Can you work these out from the model? Positions are in its coordinate system, mm. Coordinates: 2 decimals unless noted, no trailing zeros. Write each loop counter-clockwise with the first axis right and the second up, starting at its lowest first coordinate (ties: lowest second). Pieces come first, ordered by that corner, then holes. Notation, with made-up numbers: M 6,23.25 L 15,23.25 A33 cw 15,60.25 Z; hole C -11,39 d8. An arc over 180 degrees is marked long. Use one line per item in the form item = value. Start each with the question number.
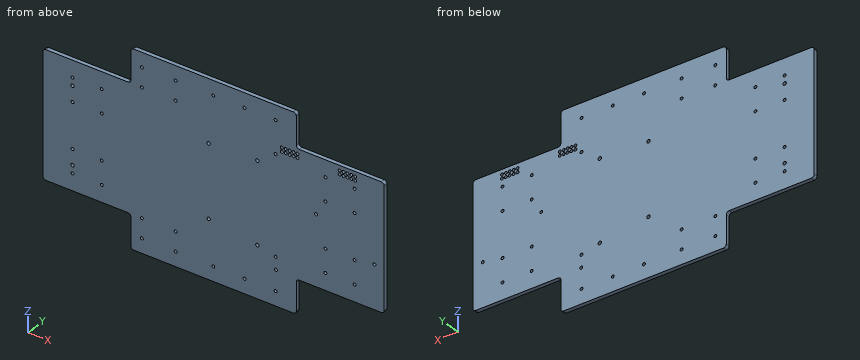
```python
from build123d import *

# Parameters (mm, degrees)
SKETCH_1_R          = 1.75
SKETCH_1_R_2        = 1.5
EXTRUDE_1_DEPTH     = 4
SKETCH_2_R          = 1.5
CUT_EXTRUDE_1_DEPTH = 5
FILLET_1_R          = 3
FILLET_2_R          = 3
FILLET_3_R          = 3
FILLET_4_R          = 3
FILLET_5_R          = 3
FILLET_6_R          = 3
FILLET_7_R          = 3
FILLET_8_R          = 3
FILLET_9_R          = 3
FILLET_10_R         = 3
FILLET_11_R         = 3
FILLET_12_R         = 3
SKETCH_3_R          = 1.75
CUT_EXTRUDE_2_DEPTH = 5
SKETCH_5_R          = 1.5
CUT_EXTRUDE_3_DEPTH = 5
SKETCH_6_R          = 1.5
CUT_EXTRUDE_4_DEPTH = 10


with BuildPart() as part:
    # 草图1 → 凸台-拉伸1 (new body)
    with BuildSketch(Plane(origin=(0, 0, 0), x_dir=(1, 0, 0), z_dir=(0, 1, 0))):
        Polygon((-165.354330709, -0.523412356), (-165.354330709, 129.476587644), (-75.154330709, 129.476587644), (-75.154330709, 164.476587644), (94.445669291, 164.476587644), (94.445669291, 129.476587644), (184.645669291, 129.476587644), (184.645669291, -0.523412356), (94.445669291, -0.523412356), (94.445669291, -35.523412356), (-75.154330709, -35.523412356), (-75.154330709, -0.523412356), align=None)
        with Locations((-135.060351007, 24.855830169)):
            Circle(SKETCH_1_R, mode=Mode.SUBTRACT)
        with Locations((-135.060351007, 104.097345119)):
            Circle(SKETCH_1_R, mode=Mode.SUBTRACT)
        with Locations((-105.060351007, 87.897345119)):
            Circle(SKETCH_1_R_2, mode=Mode.SUBTRACT)
        with Locations((-105.060351007, 112.097345119)):
            Circle(SKETCH_1_R_2, mode=Mode.SUBTRACT)
        with Locations((-135.060351007, 87.897345119)):
            Circle(SKETCH_1_R_2, mode=Mode.SUBTRACT)
        with Locations((-135.060351007, 112.097345119)):
            Circle(SKETCH_1_R_2, mode=Mode.SUBTRACT)
        with Locations((-105.060351007, 41.055830169)):
            Circle(SKETCH_1_R_2, mode=Mode.SUBTRACT)
        with Locations((-135.060351007, 41.055830169)):
            Circle(SKETCH_1_R_2, mode=Mode.SUBTRACT)
        with Locations((-105.060351007, 16.855830169)):
            Circle(SKETCH_1_R_2, mode=Mode.SUBTRACT)
        with Locations((-135.060351007, 16.855830169)):
            Circle(SKETCH_1_R_2, mode=Mode.SUBTRACT)
        with Locations((124.351689589, 16.855830169)):
            Circle(SKETCH_1_R_2, mode=Mode.SUBTRACT)
        with Locations((154.351689589, 16.855830169)):
            Circle(SKETCH_1_R_2, mode=Mode.SUBTRACT)
        with Locations((124.351689589, 41.055830169)):
            Circle(SKETCH_1_R_2, mode=Mode.SUBTRACT)
        with Locations((154.351689589, 41.055830169)):
            Circle(SKETCH_1_R_2, mode=Mode.SUBTRACT)
        with Locations((124.351689589, 87.897345119)):
            Circle(SKETCH_1_R_2, mode=Mode.SUBTRACT)
        with Locations((154.351689589, 87.897345119)):
            Circle(SKETCH_1_R_2, mode=Mode.SUBTRACT)
        with Locations((124.351689589, 112.097345119)):
            Circle(SKETCH_1_R_2, mode=Mode.SUBTRACT)
        with Locations((154.351689589, 112.097345119)):
            Circle(SKETCH_1_R_2, mode=Mode.SUBTRACT)
    extrude(amount=EXTRUDE_1_DEPTH)

    # 草图2 → 切除-拉伸1 (cut, through all)
    with BuildSketch(Plane(origin=(0, 4, 0), x_dir=(1, 0, 0), z_dir=(0, 1, 0))):
        with Locations((-29.350172185, 149.476587644)):
            Circle(SKETCH_2_R)
        with Locations((-29.350172185, 129.476587644)):
            Circle(SKETCH_2_R)
        with Locations((-63.922255051, 149.476587644)):
            Circle(SKETCH_2_R)
        with Locations((-63.922255051, 129.476587644)):
            Circle(SKETCH_2_R)
        with Locations((-29.350172185, -0.523412356)):
            Circle(SKETCH_2_R)
        with Locations((-29.350172185, -20.523412356)):
            Circle(SKETCH_2_R)
        with Locations((-63.922255051, -20.523412356)):
            Circle(SKETCH_2_R)
        with Locations((-63.922255051, -0.523412356)):
            Circle(SKETCH_2_R)
        with Locations((9.288549374, 149.476587644)):
            Circle(SKETCH_2_R)
        with Locations((41.288549374, 149.476587644)):
            Circle(SKETCH_2_R)
        with Locations((73.288549374, 149.476587644)):
            Circle(SKETCH_2_R)
        with Locations((73.288549374, 115.508346765)):
            Circle(SKETCH_2_R)
        with Locations((41.288549374, -20.523412356)):
            Circle(SKETCH_2_R)
        with Locations((73.288549374, -20.523412356)):
            Circle(SKETCH_2_R)
        with Locations((73.288549374, 13.444828523)):
            Circle(SKETCH_2_R)
        with Locations((9.288549374, -20.523412356)):
            Circle(SKETCH_2_R)
    extrude(amount=-CUT_EXTRUDE_1_DEPTH, mode=Mode.SUBTRACT)

    # 圆角1
    fillet_1_edges = [part.edges().sort_by_distance(p)[0] for p in [
        (-75.154330709, 2, -164.476587644),
    ]]
    fillet(fillet_1_edges, radius=FILLET_1_R)

    # 圆角2
    fillet_2_edges = [part.edges().sort_by_distance(p)[0] for p in [
        (-165.354330709, 2, -129.476587644),
    ]]
    fillet(fillet_2_edges, radius=FILLET_2_R)

    # 圆角3
    fillet_3_edges = [part.edges().sort_by_distance(p)[0] for p in [
        (-75.154330709, 2, -129.476587644),
    ]]
    fillet(fillet_3_edges, radius=FILLET_3_R)

    # 圆角4
    fillet_4_edges = [part.edges().sort_by_distance(p)[0] for p in [
        (-165.354330709, 2, 0.523412356),
    ]]
    fillet(fillet_4_edges, radius=FILLET_4_R)

    # 圆角5
    fillet_5_edges = [part.edges().sort_by_distance(p)[0] for p in [
        (-75.154330709, 2, 0.523412356),
    ]]
    fillet(fillet_5_edges, radius=FILLET_5_R)

    # 圆角6
    fillet_6_edges = [part.edges().sort_by_distance(p)[0] for p in [
        (-75.154330709, 2, 35.523412356),
    ]]
    fillet(fillet_6_edges, radius=FILLET_6_R)

    # 圆角7
    fillet_7_edges = [part.edges().sort_by_distance(p)[0] for p in [
        (94.445669291, 2, 35.523412356),
    ]]
    fillet(fillet_7_edges, radius=FILLET_7_R)

    # 圆角8
    fillet_8_edges = [part.edges().sort_by_distance(p)[0] for p in [
        (94.445669291, 2, 0.523412356),
    ]]
    fillet(fillet_8_edges, radius=FILLET_8_R)

    # 圆角9
    fillet_9_edges = [part.edges().sort_by_distance(p)[0] for p in [
        (184.645669291, 2, 0.523412356),
    ]]
    fillet(fillet_9_edges, radius=FILLET_9_R)

    # 圆角10
    fillet_10_edges = [part.edges().sort_by_distance(p)[0] for p in [
        (184.645669291, 2, -129.476587644),
    ]]
    fillet(fillet_10_edges, radius=FILLET_10_R)

    # 圆角11
    fillet_11_edges = [part.edges().sort_by_distance(p)[0] for p in [
        (94.445669291, 2, -129.476587644),
    ]]
    fillet(fillet_11_edges, radius=FILLET_11_R)

    # 圆角12
    fillet_12_edges = [part.edges().sort_by_distance(p)[0] for p in [
        (94.445669291, 2, -164.476587644),
    ]]
    fillet(fillet_12_edges, radius=FILLET_12_R)

    # 草图3 → 切除-拉伸2 (cut, through all)
    with BuildSketch(Plane(origin=(0, 4, 0), x_dir=(1, 0, 0), z_dir=(0, 1, 0))):
        with Locations((54.598317565, 26.976587644)):
            Circle(SKETCH_3_R)
        with Locations((54.598317565, 110.976587644)):
            Circle(SKETCH_3_R)
        with Locations((4.598317565, 28.976587644)):
            Circle(SKETCH_3_R)
        with Locations((4.598317565, 103.976587644)):
            Circle(SKETCH_3_R)
    extrude(amount=-CUT_EXTRUDE_2_DEPTH, mode=Mode.SUBTRACT)

    # 草图5 → 切除-拉伸3 (cut, through all)
    with BuildSketch(Plane(origin=(0, 4, 0), x_dir=(1, 0, 0), z_dir=(0, 1, 0))):
        with Locations((73.645669291, 128.296587644)):
            Circle(SKETCH_5_R)
        with Locations((174.645669291, 84.296587644)):
            Circle(SKETCH_5_R)
        with Locations((114.645669291, 57.296587644)):
            Circle(SKETCH_5_R)
    extrude(amount=-CUT_EXTRUDE_3_DEPTH, mode=Mode.SUBTRACT)

    # 草图6 → 切除-拉伸4 (cut)
    with BuildSketch(Plane(origin=(0, 4, 0), x_dir=(1, 0, 0), z_dir=(0, 1, 0))):
        with Locations((146.895669291, 8.486587644)):
            Circle(SKETCH_6_R)
        with Locations((83.635669291, 8.486587644)):
            Circle(SKETCH_6_R)
        with Locations((142.895669291, 8.486587644)):
            Circle(SKETCH_6_R)
        with Locations((79.635669291, 8.486587644)):
            Circle(SKETCH_6_R)
        with Locations((138.895669291, 8.486587644)):
            Circle(SKETCH_6_R)
        with Locations((87.635669291, 8.486587644)):
            Circle(SKETCH_6_R)
        with Locations((91.635669291, 8.486587644)):
            Circle(SKETCH_6_R)
        with Locations((150.895669291, 8.486587644)):
            Circle(SKETCH_6_R)
        with Locations((95.635669291, 8.486587644)):
            Circle(SKETCH_6_R)
        with Locations((154.895669291, 8.486587644)):
            Circle(SKETCH_6_R)
        with Locations((87.635669291, 4.486587644)):
            Circle(SKETCH_6_R)
        with Locations((146.895669291, 4.486587644)):
            Circle(SKETCH_6_R)
        with Locations((79.635669291, 4.486587644)):
            Circle(SKETCH_6_R)
        with Locations((83.635669291, 4.486587644)):
            Circle(SKETCH_6_R)
        with Locations((91.635669291, 4.486587644)):
            Circle(SKETCH_6_R)
        with Locations((95.635669291, 4.486587644)):
            Circle(SKETCH_6_R)
        with Locations((138.895669291, 4.486587644)):
            Circle(SKETCH_6_R)
        with Locations((142.895669291, 4.486587644)):
            Circle(SKETCH_6_R)
        with Locations((150.895669291, 4.486587644)):
            Circle(SKETCH_6_R)
        with Locations((154.895669291, 4.486587644)):
            Circle(SKETCH_6_R)
    extrude(amount=-CUT_EXTRUDE_4_DEPTH, mode=Mode.SUBTRACT)


solid = part.part
```
1) Please list where these lines run through material, in increasing order: line 1 (X direction, y = 0.55, z = 20.5); line 2 (Z direction, x = 82.5, y = 0.6); line 3 (Z direction, x = -124, y = 2.35).
2) Suppose I cut it at B-B on y = 2.9. State how many separate pieces and enclosed holes the cut face has, and give its area (3 significant figures).
3) Suppose I cut it at C-C on x = -86.5. Please give me the cut outline in (y, z).
4) Suppose I cut it at A-A on z = -137.5. Please give me the cut outline in (x, y).
5) Will these pins go through, and if not, where does the flat tip stop? pin 1 Ø1.5 at (y, z) = (1.5, -142.5) entering from -X; pin 2 Ø2 at (y, z) = (1.5, -144) entering from +X.
Computed values:
q1.line_1 = -75.15 to -65.42, -62.42 to -30.85, -27.85 to 7.79, 10.79 to 39.79, 42.79 to 71.79, 74.79 to 94.45
q1.line_2 = -164.48 to -9.47, -7.51 to -5.47, -3.51 to 35.52
q1.line_3 = -129.48 to 0.52
q2.separate_pieces = 1
q2.enclosed_holes = 61
q2.area = 56,900 mm²
q3.outline = M 0,-129.48 L 4,-129.48 L 4,0.52 L 0,0.52 Z
q4.outline = M -75.15,0 L 94.45,0 L 94.45,4 L -75.15,4 Z
q5.pin_1 = -75.15
q5.pin_2 = 94.45
